CAD build for the part. Positions are in the model's coordinates, mm. Face numbers are marked on the shaded views. A direction names the side the tool comes from. Coordinates: 2 decimals unless noted, no trailing zeros. Loops run counter-clockwise (first coordinate to the right, second up) from the corner with the lowest first, then second, coordinate; pieces in that order, holes last. Notation, with made-up numbers: (-38.75, 47) -> (-18.75, 47) arc R9 cw to (-18.75, 52) -> close; hole circle Ø7 at (-31.5, -32). An arc over 180 degrees is marked (long way). Write each question's results on one line, items separated by ' | '.
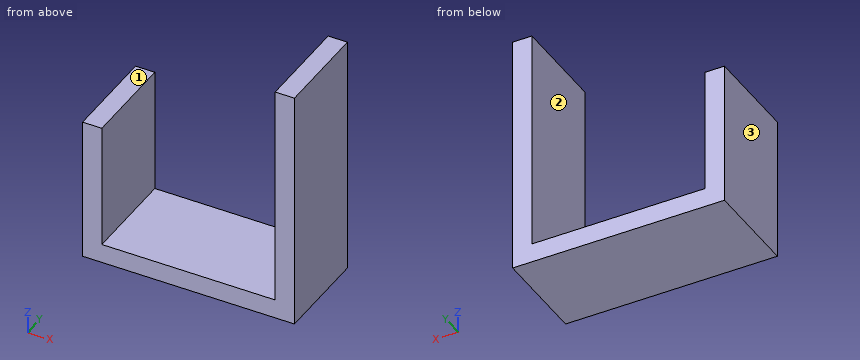
from build123d import *

# Parameters (mm, degrees)
EXTRUDE_1_DEPTH = 10


with BuildPart() as part:
    # 草圖1 → 填料-伸長1 (new body)
    with BuildSketch(Plane(origin=(0, 0, 0), x_dir=(1, 0, 0), z_dir=(0, 1, 0))):
        Polygon((-10, -7.5), (-8, -7.5), (-8, 5.5), (10, 5.5), (10, -17.760223048), (12, -17.760223048), (12, 7.5), (10, 7.5), (-10, 7.5), align=None)
    extrude(amount=EXTRUDE_1_DEPTH)


solid = part.part
1) Drill centre lines: L1, parallel to X at y = 7.75, z = -4.5; L2, parallel to X at y = 8.25, z = 8.5; L3, parallel to Z at x = -5, y = 7.5. Where is each one in solid material? Low to high. Write a range as from..to.
Outcome:
L1: x = -10..-8, 10..12 | L2: x = 10..12 | L3: z = -7.5..-5.5
2) Slice it at D-D (x = 7). Write the cut outline in (y, z), then the cut area to 3 significant figures.
Outcome:
outline: (0, -7.5) -> (10, -7.5) -> (10, -5.5) -> (0, -5.5) -> close | area: 20.0 mm^2
3) Which spindle directions (+Z, -Z, +X, -X, +Y, -Y) get a long thin tool onto all of the face, cutting with end or side? Do the marked faces 1, 2 and 3. Say none if no direction does.
Outcome:
face 1: +Z, -X, +Y, -Y | face 2: +Z, +Y, -Y | face 3: +Z, -Z, -X, +Y, -Y
4) Slice it at C-C (z = 13.75). Write the cut outline in (x, y).
Outcome:
outline: (10, 0) -> (12, 0) -> (12, 10) -> (10, 10) -> close
5) Slice it at A-A (z = 3.5). Write the cut outline in (x, y), then the cut area to 3 significant figures.
Outcome:
outline: (-10, 0) -> (-8, 0) -> (-8, 10) -> (-10, 10) -> close; (10, 0) -> (12, 0) -> (12, 10) -> (10, 10) -> close | area: 40.0 mm^2
6) Slice it at B-B (y = 8.5). Write the cut outline in (x, z), then the cut area to 3 significant figures.
Outcome:
outline: (-10, -7.5) -> (12, -7.5) -> (12, 17.76) -> (10, 17.76) -> (10, -5.5) -> (-8, -5.5) -> (-8, 7.5) -> (-10, 7.5) -> close | area: 117 mm^2
7) Pin check, flat tips, straight feed: pin 1 (1.6 mm diameter, centred on x = -9, y = 6, fed in from +Z); pin 2 (4 mm diameter, centred on x = 5.5, y = 2, fed in from +Z). Stop position of each tip, or through.
Outcome:
pin 1: stops at z = 7.5 | pin 2: stops at z = -5.5
